Here's how the part is built. I have some questions about the finished solid (model axes, mm). Face numbers are marked on the shaded views. Coordinates: 2 decimals unless noted, no trailing zeros. Order: outer loops, then holes, each group sorted by start corner. A loop starts at its lowest first (then second) coordinate and runs counter-clockwise, first axis right, second up.
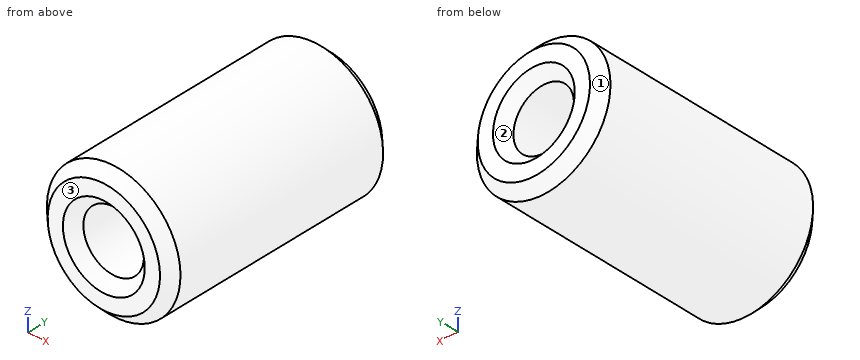
```python
from build123d import *

# Parameters (mm, degrees)
SKETCH1_R           = 22.5
BOSS_EXTRUDE1_DEPTH = 81.030916
SKETCH2_R           = 10.199174828
CUT_EXTRUDE1_DEPTH  = 88.05463427
CHAMFER1_SIZE       = 3.590257
CHAMFER1_SIZE_2     = 3.580234


with BuildPart() as part:
    # Sketch1 → Boss-Extrude1 (new body)
    with BuildSketch(Plane(origin=(0, 0, 0), x_dir=(1, 0, 0), z_dir=(0, 1, 0))):
        with Locations(Location((0, 0, 0), (0, 0, 270))):
            Circle(SKETCH1_R)
    extrude(amount=BOSS_EXTRUDE1_DEPTH)

    # Sketch2 → Cut-Extrude1 (cut, through all)
    with BuildSketch(Plane(origin=(0, 0, 0), x_dir=(1, 0, 0), z_dir=(0, 1, 0))):
        with Locations(Location((0, 0, 0), (0, 0, 270))):
            Circle(SKETCH2_R)
    extrude(amount=CUT_EXTRUDE1_DEPTH, mode=Mode.SUBTRACT)

    # Chamfer1
    # the kernel refuses this chamfer: 3.590257, 3.580234 mm, written as the material it takes off along each edge
    with BuildSketch(Plane(origin=(0, 0, 0), x_dir=(0, 0, 1), z_dir=(-1, 0, 0))) as chamfer1_piece_1:
        Polygon((22.5, CHAMFER1_SIZE), (22.5 - CHAMFER1_SIZE_2, 0), (22.5, 0), align=None)
    revolve(axis=Axis((0, 0, 0), (0, 1, 0)), mode=Mode.SUBTRACT)
    with BuildSketch(Plane(origin=(0, 81.030916, 0), x_dir=(0, 0, 1), z_dir=(-1, 0, 0))) as chamfer1_piece_2:
        Polygon((22.5, -CHAMFER1_SIZE_2), (22.5 - CHAMFER1_SIZE, 0), (22.5, 0), align=None)
    revolve(axis=Axis((0, 81.030916, 0), (0, 1, 0)), mode=Mode.SUBTRACT)
    with BuildSketch(Plane(origin=(0, 0, 0), x_dir=(0, 0, 1), z_dir=(-1, 0, 0))) as chamfer1_piece_3:
        Polygon((10.199174828 + CHAMFER1_SIZE, 0), (10.199174828, CHAMFER1_SIZE_2), (10.199174828, 0), align=None)
    revolve(axis=Axis((0, 0, 0), (0, 1, 0)), mode=Mode.SUBTRACT)
    with BuildSketch(Plane(origin=(0, 81.030916, 0), x_dir=(0, 0, 1), z_dir=(1, 0, 0))) as chamfer1_piece_4:
        Polygon((10.199174828 + CHAMFER1_SIZE_2, 0), (10.199174828, CHAMFER1_SIZE), (10.199174828, 0), align=None)
    revolve(axis=Axis((0, 81.030916, 0), (0, -1, 0)), mode=Mode.SUBTRACT)


solid = part.part
```
Q1. If we section it at B-B on x = 0: Write out the boundary of the cut face in (y, z).
Q2. We'd pull the mould along X, two halves only. Please class the marked faces 1, 2 and 3: pulls with the +X half, pulls with the -X half, needs draft (parallel to the pull), parting line crosses it, or undercut.
Q3. If we section it at A-A on z = 0: Write out the boundary of the cut face in (x, y).
Q4. Will these pins go through, and if not, where does the flat tip stop? pin 1 (3 mm diameter, centred on x = -15.5, y = 14, fed in from +Z); pin 2 (12 mm diameter, centred on y = 27, z = -4.5, fed in from -X); pin 3 (6 mm diameter, centred on y = 24, z = -10.5, fed in from -X).
Q5. I need wall thicknesses on L1, parallel to X at y = 18, z = 0; L2, parallel to X at y = 23, z = -9; L3, parallel to Z at x = 2, y = 7.5. Which ranges of each line are inside material? Lowest first, please.
Q6. If we section it at C-C on y = 54: Write out the boundary of the cut face in (x, z), then the cut area to 3 significant figures.
Reply:
1. outline: (0, -18.92) - (3.59, -22.5) - (77.45, -22.5) - (81.03, -18.91) - (81.03, -13.78) - (77.44, -10.2) - (3.58, -10.2) - (0, -13.79) - close; (0, 13.79) - (3.58, 10.2) - (77.44, 10.2) - (81.03, 13.78) - (81.03, 18.91) - (77.45, 22.5) - (3.59, 22.5) - (0, 18.92) - close
2. face 1: parting line crosses it
2. face 2: undercut
2. face 3: needs draft
3. outline: (-22.5, 3.59) - (-18.92, 0) - (-13.79, 0) - (-10.2, 3.58) - (-10.2, 77.44) - (-13.78, 81.03) - (-18.91, 81.03) - (-22.5, 77.45) - close; (10.2, 3.58) - (13.79, 0) - (18.92, 0) - (22.5, 3.59) - (22.5, 77.45) - (18.91, 81.03) - (13.78, 81.03) - (10.2, 77.44) - close
4. pin 1: stops at z = 17.61
4. pin 2: stops at x = -22.5
4. pin 3: stops at x = -21.21
5. L1: x = -22.5 to -10.2, 10.2 to 22.5
5. L2: x = -20.62 to -4.8, 4.8 to 20.62
5. L3: z = -22.41 to -10, 10 to 22.41
6. outline: circle Ø45 at (0, 0); hole circle Ø20.4 at (0, 0)
6. area: 1,260 mm2
